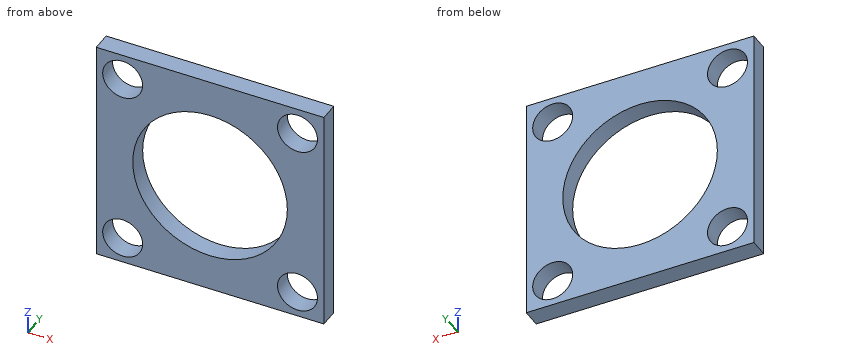
```python
from build123d import *

# Parameters (mm, degrees)
ESQUISSE1_W             = 6
ESQUISSE1_H             = 6
EXTRUSION1_DEPTH        = 0.5
ESQUISSE2_R             = 2.037099296
ENL_V_MAT_EXTRU_1_DEPTH = 1.5
ESQUISSE3_R             = 0.526608141
ENL_V_MAT_EXTRU_3_DEPTH = 1.5


with BuildPart() as part:
    # Esquisse1 → Extrusion1 (new body)
    with BuildSketch(Plane(origin=(0, 0, 0), x_dir=(1, 0, 0), z_dir=(0, 1, 0))):
        with Locations((3, 3)):
            Rectangle(ESQUISSE1_W, ESQUISSE1_H)
    extrude(amount=EXTRUSION1_DEPTH)

    # Esquisse2 → Enlèv. mat.-Extru.1 (cut, through all)
    with BuildSketch(Plane(origin=(0, 0.5, 0), x_dir=(-1, 0, 0), z_dir=(0, 1, 0))):
        with Locations(Location((-3, -3, 0), (0, 0, 90))):  # turned: the seam where the file's is
            Circle(ESQUISSE2_R)
    extrude(amount=-ENL_V_MAT_EXTRU_1_DEPTH, mode=Mode.SUBTRACT)

    # Esquisse3 → Enlèv. mat.-Extru.3 (cut, through all)
    with BuildSketch(Plane(origin=(0, 0.5, 0), x_dir=(-1, 0, 0), z_dir=(0, 1, 0))):
        with Locations(Location((-0.695868946, -5.304131054, 0), (0, 0, 90))):  # turned: the seam where the file's is
            Circle(ESQUISSE3_R)
        with Locations(Location((-5.304131054, -5.304131054, 0), (0, 0, 90))):  # turned: the seam where the file's is
            Circle(ESQUISSE3_R)
        with Locations(Location((-5.304131054, -0.695868946, 0), (0, 0, 90))):  # turned: the seam where the file's is
            Circle(ESQUISSE3_R)
        with Locations(Location((-0.695868946, -0.695868946, 0), (0, 0, 90))):  # turned: the seam where the file's is
            Circle(ESQUISSE3_R)
    extrude(amount=-ENL_V_MAT_EXTRU_3_DEPTH, mode=Mode.SUBTRACT)


solid = part.part
```
Input: part model. Units: mm. Frame: model coordinates. Coordinates: 2 decimals unless noted, no trailing zeros. Loops run counter-clockwise (first coordinate to the right, second up) from the corner with the lowest first, then second, coordinate; pieces in that order, holes last. Notation, with made-up numbers: M 85,-12.75 L 90,-12.75 A16 ccw 90,7.25 Z; hole C 73,-23 d7. An arc over 180 degrees is marked long. Use a Markdown table: item, result. Add a question column.
1) Section B-B, the plane z = -3. Return the cut outline in (x, y).
2) Section C-C, the plane y = 0.25. Return the cut outline in (x, z).
3) Section A-A, the plane x = 3. Return the cut outline in (y, z), plus the area to 3 significant figures.
4) Pin query (flat end, axial travel): P1, Ø1.4, axis at x = 5.3, z = -0.7, coming from the -Y side. Return the tip coordinate at first contact, or that it passes through.
5) Line query: L1, parallel to X at y = 0.25, z = -0.5; L2, parallel to X at y = 0.3, z = -0.4; L3, parallel to Z at x = 0.9, y = 0.2. Output: solid intervals per line, ascending. Write a range as from..to.
6) Section D-D, the plane z = -5.15. Return the cut outline in (x, y), plus the area to 3 significant figures.
Answer below:
| question | item | result |
|---|---|---|
| 1 | outline | M 0,0 L 0.96,0 L 0.96,0.5 L 0,0.5 Z; M 5.04,0 L 6,0 L 6,0.5 L 5.04,0.5 Z |
| 2 | outline | M 0,-6 L 6,-6 L 6,0 L 0,0 Z; hole C 0.7,-5.3 d1.05; hole C 0.7,-0.7 d1.05; hole C 3,-3 d4.07; hole C 5.3,-5.3 d1.05; hole C 5.3,-0.7 d1.05 |
| 3 | outline | M 0,-6 L 0.5,-6 L 0.5,-5.04 L 0,-5.04 Z; M 0,-0.96 L 0.5,-0.96 L 0.5,0 L 0,0 Z |
| 3 | area | 0.963 mm2 |
| 4 | P1 | y = 0 |
| 5 | L1 | 0..0.21, 1.18..4.82, 5.79..6 |
| 5 | L2 | 0..0.26, 1.13..4.87, 5.74..6 |
| 5 | L3 | -6..-5.79, -4.82..-1.18, -0.21..0 |
| 6 | outline | M 0,0 L 0.19,0 L 0.19,0.5 L 0,0.5 Z; M 1.2,0 L 4.8,0 L 4.8,0.5 L 1.2,0.5 Z; M 5.81,0 L 6,0 L 6,0.5 L 5.81,0.5 Z |
| 6 | area | 1.99 mm2 |
